Check sheet for the modelled part. Datum: model origin and axes. Units: mm. A direction names the side the tool comes from. Round coordinates to 2 decimals unless told otherwise and drop trailing zeros. Order: outer loops, then holes, each group sorted by start corner. A loop starts at its lowest first (then second) coordinate and runs counter-clockwise, first axis right, second up. Notation, with made-up numbers: (76, 4.5) -> (97, 4.5) arc R19 ccw to (97, 39.5) -> close; hole circle Ø8 at (-33, 17.5). An arc over 180 degrees is marked (long way). Answer in a Markdown table with one row per item.
```python
from build123d import *

# Parameters (mm, degrees)
SKETCH1_W               = 67.5
SKETCH1_H               = 35.5
SKETCH1_W_2             = 62.5
SKETCH1_H_2             = 30.5
BOSS_EXTRUDE1_DEPTH     = 1
SKETCH2_W               = 67.5
SKETCH2_H               = 35.5
SKETCH2_W_2             = 60.5
SKETCH2_H_2             = 28.5
BOSS_EXTRUDE2_DEPTH     = 0.5
SKETCH3_R               = 3.535533906
BOSS_EXTRUDE3_DEPTH     = 1.5
SKETCH4_R               = 0.75
CUT_EXTRUDE1_DEPTH      = 1
CUT_EXTRUDE1_DEPTH_BACK = 2.5


with BuildPart() as part:
    # Sketch1 → Boss-Extrude1 (new body)
    with BuildSketch(Plane(origin=(0, 0, 0), x_dir=(1, 0, 0), z_dir=(0, 1, 0))):
        Rectangle(SKETCH1_W, SKETCH1_H)
        Rectangle(SKETCH1_W_2, SKETCH1_H_2, mode=Mode.SUBTRACT)
    extrude(amount=BOSS_EXTRUDE1_DEPTH)

    # Sketch2 → Boss-Extrude2 (add)
    with BuildSketch(Plane.XZ):
        Rectangle(SKETCH2_W, SKETCH2_H)
        Rectangle(SKETCH2_W_2, SKETCH2_H_2, mode=Mode.SUBTRACT)
    extrude(amount=BOSS_EXTRUDE2_DEPTH)

    # Sketch3 → Boss-Extrude3 (add)
    with BuildSketch(Plane(origin=(0, 1, 0), x_dir=(1, 0, 0), z_dir=(0, 1, 0))):
        with Locations((-33.75, 17.75)):
            Circle(SKETCH3_R)
        with Locations((33.75, 17.75)):
            Circle(SKETCH3_R)
        with Locations((33.75, -17.75)):
            Circle(SKETCH3_R)
        with Locations((-33.75, -17.75)):
            Circle(SKETCH3_R)
        with BuildLine():
            Line((-3.535533906, 17.75), (3.535533906, 17.75))
            ThreePointArc((3.535533906, 17.75), (0, 21.285533906), (-3.535533906, 17.75))
        make_face()
        with BuildLine():
            Line((-3.535533906, -17.75), (3.535533906, -17.75))
            ThreePointArc((3.535533906, -17.75), (0, -21.285533906), (-3.535533906, -17.75))
        make_face()
    extrude(amount=-BOSS_EXTRUDE3_DEPTH)

    # Sketch4 → Cut-Extrude1 (cut, two sides)
    with BuildSketch(Plane(origin=(0, 1, 0), x_dir=(1, 0, 0), z_dir=(0, 1, 0))) as cut_extrude1_sk:
        with Locations((-33.75, 17.75)):
            Circle(SKETCH4_R)
        with Locations((33.75, 17.75)):
            Circle(SKETCH4_R)
        with Locations((33.75, -17.75)):
            Circle(SKETCH4_R)
        with Locations((-33.75, -17.75)):
            Circle(SKETCH4_R)
        with Locations((0, 17.75)):
            Circle(SKETCH4_R)
        with Locations((0, -17.75)):
            Circle(SKETCH4_R)
    extrude(amount=CUT_EXTRUDE1_DEPTH, mode=Mode.SUBTRACT)
    extrude(cut_extrude1_sk.sketch, amount=-CUT_EXTRUDE1_DEPTH_BACK, mode=Mode.SUBTRACT)


solid = part.part
```
(1) Draft check along Z on faces 1 (the flat face through (0, 0, 15)), 2 (the cylindrical face through (0.078, 0.26, -21.285)), 3 (the flat face through (17, 0, 17.75)). Enter one of: pulls with the +Z half, pulls with the -Z half, needs draft (parallel to the pull), parting line crosses it, or undercut.
Solutions:
| item | result |
|---|---|
| face 1 | undercut |
| face 2 | pulls with the -Z half |
| face 3 | pulls with the +Z half |
(2) Tool access check on faces 4 (the flat face through (17, 0, -17.75)), 5 (the flat face through (-33.75, 0, 0)), 6 (the flat face through (-17, 0, 17.75)), 7 (the flat face through (33.75, 0, 0)). Record the directions out of +Z, -Z, +X, -X, +Y, -Y that give a thin tool (end or side, any length) a straight path to the whole face; none if there is none.
Solutions:
| item | result |
|---|---|
| face 4 | -Z, +Y, -Y |
| face 5 | -X, +Y, -Y |
| face 6 | +Z, +Y, -Y |
| face 7 | +X, +Y, -Y |
(3) Section check A-A on z = -13. Record the boundary of the cut face in (x, y), plus the area to 3 significant figures.
Solutions:
| item | result |
|---|---|
| outline | (-33.75, -0.5) -> (-30.25, -0.5) -> (-30.25, 0) -> (-31.25, 0) -> (-31.25, 1) -> (-33.75, 1) -> close; (30.25, -0.5) -> (33.75, -0.5) -> (33.75, 1) -> (31.25, 1) -> (31.25, 0) -> (30.25, 0) -> close |
| area | 8.50 mm^2 |
(4) Section check C-C on y = 0.4. Record the boundary of the cut face in (x, z), plus the area to 3 significant figures.
Solutions:
| item | result |
|---|---|
| outline | (-33.75, -14.21) arc R3.54 ccw (long way) to (-30.21, -17.75) -> (-3.54, -17.75) arc R3.54 ccw to (3.54, -17.75) -> (30.21, -17.75) arc R3.54 ccw (long way) to (33.75, -14.21) -> (33.75, 14.21) arc R3.54 ccw (long way) to (30.21, 17.75) -> (3.54, 17.75) arc R3.54 ccw to (-3.54, 17.75) -> (-30.21, 17.75) arc R3.54 ccw (long way) to (-33.75, 14.21) -> close; hole circle Ø1.5 at (-33.75, -17.75); hole circle Ø1.5 at (-33.75, 17.75); hole (-31.25, -15.25) -> (31.25, -15.25) -> (31.25, 15.25) -> (-31.25, 15.25) -> close; hole circle Ø1.5 at (0, -17.75); hole circle Ø1.5 at (0, 17.75); hole circle Ø1.5 at (33.75, -17.75); hole circle Ø1.5 at (33.75, 17.75) |
| area | 636 mm^2 |
(5) Depth check by flat-ended pin: pin 1 Ø0.8 at (y, z) = (0.5, -7.5) entering from -X; pin 2 Ø0.8 at (x, y) = (-8, 0.5) entering from +Z; pin 3 Ø5 at (x, z) = (-26.5, -7.5) entering from -Y; pin 4 Ø0.6 at (y, z) = (-0.5, -3.5) entering from +X. Enter the tip coordinate at first touch or a pass-through.
Solutions:
| item | result |
|---|---|
| pin 1 | x = -33.75 |
| pin 2 | z = 17.75 |
| pin 3 | through |
| pin 4 | x = 33.75 |
(6) Section check D-D on x = 14.5. Record the boundary of the cut face in (y, z).
Solutions:
| item | result |
|---|---|
| outline | (-0.5, -17.75) -> (1, -17.75) -> (1, -15.25) -> (0, -15.25) -> (0, -14.25) -> (-0.5, -14.25) -> close; (-0.5, 14.25) -> (0, 14.25) -> (0, 15.25) -> (1, 15.25) -> (1, 17.75) -> (-0.5, 17.75) -> close |
(7) Section check B-B on x = 0. Record the boundary of the cut face in (y, z), plus the area to 3 significant figures.
Solutions:
| item | result |
|---|---|
| outline | (-0.5, -21.29) -> (1, -21.29) -> (1, -18.5) -> (-0.5, -18.5) -> close; (-0.5, -17) -> (1, -17) -> (1, -15.25) -> (0, -15.25) -> (0, -14.25) -> (-0.5, -14.25) -> close; (-0.5, 14.25) -> (0, 14.25) -> (0, 15.25) -> (1, 15.25) -> (1, 17) -> (-0.5, 17) -> close; (-0.5, 18.5) -> (1, 18.5) -> (1, 21.29) -> (-0.5, 21.29) -> close |
| area | 14.6 mm^2 |
(8) Scan lines: probe 1 along Z at (x, y) = (0, 0.6); probe 2 along X at (y, z) = (0.7, 6.5); probe 3 along Z at (x, y) = (22, 0.7). Record each from-to range of solid material in increasing order. Write a range as from..to.
Solutions:
| item | result |
|---|---|
| probe 1 | -21.29..-18.5, -17..-15.25, 15.25..17, 18.5..21.29 |
| probe 2 | -33.75..-31.25, 31.25..33.75 |
| probe 3 | -17.75..-15.25, 15.25..17.75 |
